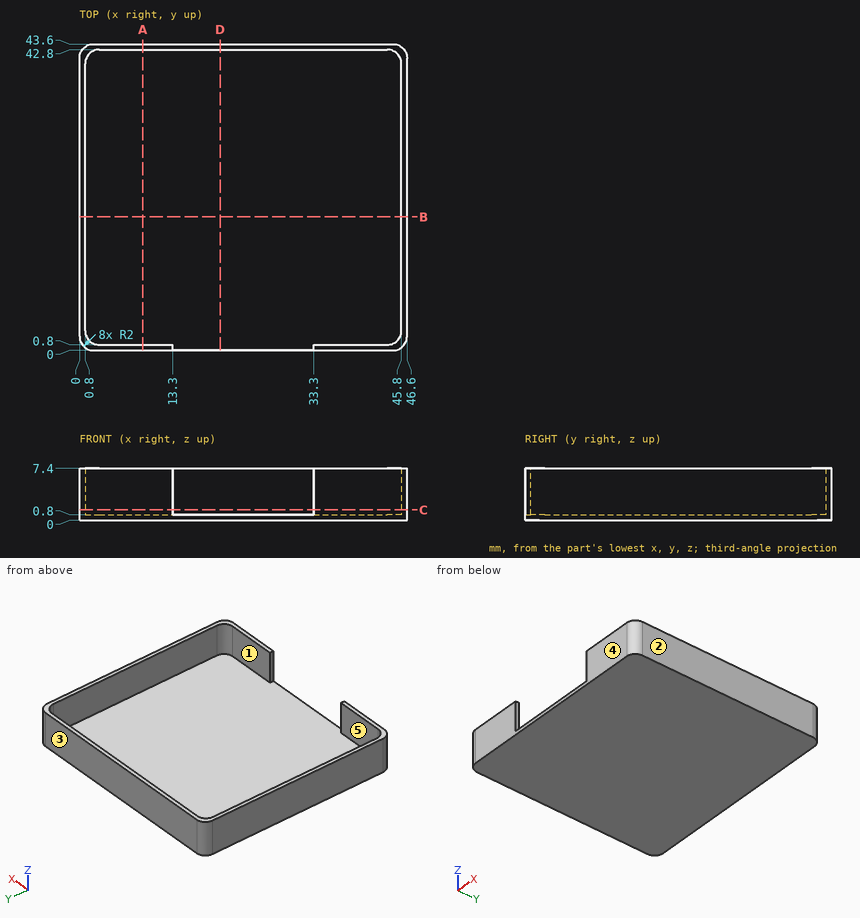
Input: dimensioned drawing with shaded views. Units: mm. Origin: part minimum x, y, z. A direction names the side the tool comes from. Give positions to 0.01 mm unless a question says otherwise; leave off trailing zeros. Order: outer loops, then holes, each group sorted by start corner. A loop starts at its lowest first (then second) coordinate and runs counter-clockwise, first axis right, second up.
(1) Pull-direction query (Y, two-part tool) for the marked faces 1, 2 and 3; classes: +Y half, -Y half, draft (parallel to the pull), parting line (faces both ways), or undercut.
(2) Access query for the marked faces 4 and 5. Directions: +Z, -Z, +X, -X, +Y, -Y. A direction counts if a zero-diameter tool reaches every point of the face in a straight line with its end or side. Return the directions, or none.
(3) Contact query for flat-ended pins moving along their axis: P1, Ø0.9, axis at y = 0.5, z = 4.5, coming from the -X side; P2, Ø0.6, axis at y = 0.5, z = 3.5, coming from the +X side. Output: stop coordinate, or through.
(4) Section query A-A (x = 9). Return the cut outline in (y, z).
(5) Material intervals for line 1 along Y through (x, z) = (3, 6); line 2 along X through (y, z) = (35, 1.5); line 3 along Y through (x, z) = (29, 2.5), sorted ascending.
(6) Section query D-D (x = 20). Return the cut outline in (y, z).
(7) Section query C-C (z = 1.5). Return the cut outline in (x, y).
(8) Section query B-B (y = 19). Return the cut outline in (x, z), plus the area to 3 significant figures.
Outcome:
1. face 1: undercut
1. face 2: draft
1. face 3: +Y half
2. face 4: +Z, -Z, +X, -X, -Y
2. face 5: +Z
3. P1: stops at x = 0.3
3. P2: stops at x = 46.2
4. outline: (0, 0) - (43.6, 0) - (43.6, 7.4) - (42.8, 7.4) - (42.8, 0.8) - (0.8, 0.8) - (0.8, 7.4) - (0, 7.4) - close
5. line 1: y = 0 to 0.8, 42.8 to 43.6
5. line 2: x = 0 to 0.8, 45.8 to 46.6
5. line 3: y = 42.8 to 43.6
6. outline: (0, 0) - (43.6, 0) - (43.6, 7.4) - (42.8, 7.4) - (42.8, 0.8) - (0, 0.8) - close
7. outline: (0, 2) arc R2 ccw to (2, 0) - (13.3, 0) - (13.3, 0.8) - (2.8, 0.8) arc R2 cw to (0.8, 2.8) - (0.8, 40.8) arc R2 cw to (2.8, 42.8) - (43.8, 42.8) arc R2 cw to (45.8, 40.8) - (45.8, 2.8) arc R2 cw to (43.8, 0.8) - (33.3, 0.8) - (33.3, 0) - (44.6, 0) arc R2 ccw to (46.6, 2) - (46.6, 41.6) arc R2 ccw to (44.6, 43.6) - (2, 43.6) arc R2 ccw to (0, 41.6) - close
8. outline: (0, 0) - (46.6, 0) - (46.6, 7.4) - (45.8, 7.4) - (45.8, 0.8) - (0.8, 0.8) - (0.8, 7.4) - (0, 7.4) - close
8. area: 47.8 mm2
